Input: part model. Units: mm. Frame: model coordinates. Face numbers are marked on the shaded views. A direction names the side the tool comes from. Round coordinates to 2 decimals unless told otherwise and drop trailing zeros. Order: outer loops, then holes, each group sorted by start corner. A loop starts at its lowest first (then second) coordinate and runs counter-clockwise, first axis right, second up. Notation, with made-up numbers: (-8, 35) -> (47, 35) arc R27 cw to (47, 63) -> close; hole circle Ø9 at (33.25, -32.5). An arc over 180 degrees is marked (long way). Answer as CSV lines item,"result". Start each with the question number.
1) Section query A-A, the plane x = 46.5. Output: boundary loops of the cut face in (y, z).
2) Mould query, pull axis Y, two halves, no side actions, for the marked faces 1, 2, 3 and 4. Classes: +Y half, -Y half, draft (parallel to the pull), parting line (faces both ways), or undercut.
3) Section query B-B, the plane z = 12.7. State how many separate pieces and enclosed holes the cut face has, and give its area (3 significant figures).
4) Line query: L1, parallel to Y at x = 77, z = 23.75; L2, parallel to X at y = 45.25, z = 12.7; L3, parallel to X at y = 45.95, z = 12.7. Output: solid intervals per line, ascending.
5) Section query C-C, the plane y = 79.5. Output: boundary loops of the cut face in (x, z), and give its area (3 significant figures).
6) First-contact query: P1, Ø1.5, axis at y = 92, z = 10, coming from the +X side; P2, Ø10, axis at x = -4, z = 11, coming from the +Y side; P3, Ø1.5, axis at y = 54.5, z = 14.5, coming from the -X side. Flat tips, straight axial feed; report the tip coordinate or a pass-through.
7) Access query for the marked faces 5, 6 and 7. Directions: +Z, -Z, +X, -X, +Y, -Y. A direction counts if a zero-diameter tool reaches every point of the face in a straight line with its end or side. Return the directions, or none.
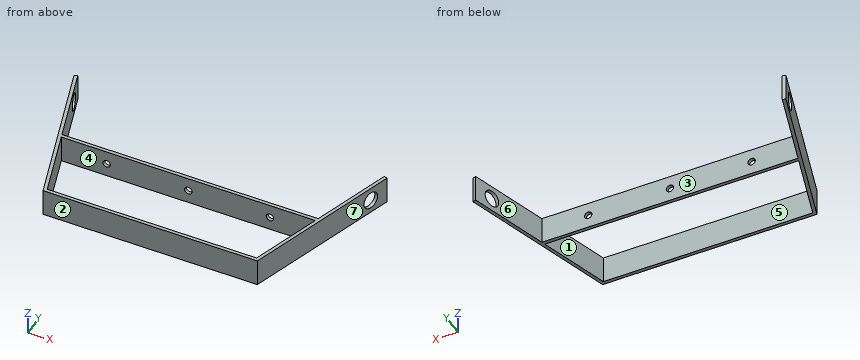
```python
from build123d import *

# Parameters (mm, degrees)
BOSS_EXTRUDE1_DEPTH = 25.4
SKETCH2_R           = 7.9375
CUT_EXTRUDE1_DEPTH  = 25.4
SKETCH3_R           = 7.9375
CUT_EXTRUDE2_DEPTH  = 25.4
BOSS_EXTRUDE2_DEPTH = 25.4
SKETCH6_R           = 3.457615734
CUT_EXTRUDE4_DEPTH  = 3.175


with BuildPart() as part:
    # Sketch1 → Boss-Extrude1 (new body)
    with BuildSketch(Plane.XY):
        Polygon((-95.914729745, -24.450906393), (104.110270255, -24.450906393), (150.147770255, 120.829197523), (147.121101424, 121.788312106), (101.785788593, -21.275906393), (-93.590248082, -21.275906393), (-138.925560913, 121.788312106), (-141.952229745, 120.829197523), align=None)
    extrude(amount=BOSS_EXTRUDE1_DEPTH)

    # Sketch2 → Cut-Extrude1 (cut)
    with BuildSketch(Plane(origin=(-94.203233113, -29.851860148, 0), x_dir=(0, 0, 1), z_dir=(-0.953281522, -0.302083333, 0))):
        with Locations((12.7, 139.015644022)):
            Circle(SKETCH2_R)
    extrude(amount=-CUT_EXTRUDE1_DEPTH, mode=Mode.SUBTRACT)

    # Sketch3 → Cut-Extrude2 (cut)
    with BuildSketch(Plane(origin=(101.650894981, -32.211933717, 0), x_dir=(0, 0, -1), z_dir=(0.953281522, -0.302083333, 0))):
        with Locations((-12.7, 141.491380218)):
            Circle(SKETCH3_R)
    extrude(amount=-CUT_EXTRUDE2_DEPTH, mode=Mode.SUBTRACT)

    # Sketch5 → Boss-Extrude2 (add)
    with BuildSketch(Plane(origin=(0, 0, 0), x_dir=(-1, 0, 0), z_dir=(0, 0, -1))):
        Polygon((-123.641976424, 47.695459109), (115.446435913, 47.695459109), (114.440316985, 44.520459109), (-122.635857495, 44.520459109), align=None)
    extrude(amount=-BOSS_EXTRUDE2_DEPTH)

    # Sketch6 → Cut-Extrude4 (cut)
    with BuildSketch(Plane(origin=(0, 47.695459109, 0), x_dir=(1, 0, 0), z_dir=(0, 1, 0))):
        with Locations((-72.103023576, -12.7)):
            Circle(SKETCH6_R)
        with Locations((4.096976424, -12.7)):
            Circle(SKETCH6_R)
        with Locations((80.296976424, -12.7)):
            Circle(SKETCH6_R)
    extrude(amount=-CUT_EXTRUDE4_DEPTH, mode=Mode.SUBTRACT)


solid = part.part
```
Findings:
1,outline,"(-24.45, 0) -> (-21.28, 0) -> (-21.28, 25.4) -> (-24.45, 25.4) -> close; (44.52, 0) -> (47.7, 0) -> (47.7, 25.4) -> (44.52, 25.4) -> close"
2,face 1,"undercut"
2,face 2,"-Y half"
2,face 3,"+Y half"
2,face 4,"undercut"
3,separate pieces,"5"
3,enclosed holes,"0"
3,area,"2,180 mm^2"
4,L1,"y = -24.45 to -21.28, 44.52 to 47.7"
4,L2,"x = -118 to -75.56, -68.65 to 0.64, 7.55 to 76.84, 83.75 to 126.2"
4,L3,"x = -118.22 to -75.56, -68.65 to 0.64, 7.55 to 76.84, 83.75 to 126.42"
5,outline,"(-128.86, 0) -> (-125.52, 0) -> (-125.52, 25.4) -> (-128.86, 25.4) -> close; (133.72, 0) -> (137.05, 0) -> (137.05, 25.4) -> (133.72, 25.4) -> close"
5,area,"169 mm^2"
6,P1,"stops at x = 141.25"
6,P2,"stops at y = 47.7"
6,P3,"stops at x = -121.17"
7,face 5,"+Z, -Z"
7,face 6,"+Z, -Z, +Y"
7,face 7,"+Z, -Z, +X, -Y"
